Input: part model. Units: mm. Frame: model coordinates. A direction names the side the tool comes from. Coordinates: 2 decimals unless noted, no trailing zeros. Order: outer loops, then holes, each group sorted by start corner. A loop starts at its lowest first (then second) coordinate and runs counter-clockwise, first axis right, second up. Notation, with made-up numbers: (-19.5, -20) - (19.5, -20) arc R18 ccw to (19.5, 2) - close; hole circle Ø1 at (89, 45.25). An arc over 180 degrees is marked (long way). Use a Markdown table: item, result. Add a question column.
from build123d import *

# Parameters (mm, degrees)
SKETCH1_R           = 2.4892
BOSS_EXTRUDE1_DEPTH = 2.286
FILLET1_R           = 5.08


with BuildPart() as part:
    # Sketch1 → Boss-Extrude1 (new body)
    with BuildSketch(Plane.XY):
        with BuildLine():
            ThreePointArc((-10.16, 0), (-8.672102448, -3.592102448), (-5.08, -5.08))
            Line((-5.08, -5.08), (30.48, -5.08))
            ThreePointArc((30.48, -5.08), (34.072102448, -3.592102448), (35.56, 0))
            Line((35.56, 0), (35.56, 279.0825))
            ThreePointArc((35.56, 279.0825), (34.072102448, 282.674602448), (30.48, 284.1625))
            Line((30.48, 284.1625), (-5.08, 284.1625))
            ThreePointArc((-5.08, 284.1625), (-8.672102448, 282.674602448), (-10.16, 279.0825))
            Line((-10.16, 279.0825), (-10.16, 0))
        make_face()
        Circle(SKETCH1_R, mode=Mode.SUBTRACT)
        with BuildLine():
            Line((9.702242909, 36.253036461), (20.782825554, 11.949932204))
            ThreePointArc((20.782825554, 11.949932204), (20.433295811, 7.094715037), (16.160582646, 4.7625))
            Line((16.160582646, 4.7625), (5.08, 4.7625))
            ThreePointArc((5.08, 4.7625), (1.487897552, 6.250397552), (0, 9.8425))
            Line((0, 9.8425), (0, 34.145604258))
            ThreePointArc((0, 34.145604258), (4.001712927, 39.109846092), (9.702242909, 36.253036461))
        make_face(mode=Mode.SUBTRACT)
        with BuildLine():
            Line((0, 107.618145742), (0, 131.92125))
            ThreePointArc((0, 131.92125), (1.487897552, 135.513352448), (5.08, 137.00125))
            Line((5.08, 137.00125), (16.160582646, 137.00125))
            ThreePointArc((16.160582646, 137.00125), (20.433295811, 134.669034963), (20.782825554, 129.813817796))
            Line((20.782825554, 129.813817796), (9.702242909, 105.510713539))
            ThreePointArc((9.702242909, 105.510713539), (4.001712927, 102.653903908), (0, 107.618145742))
        make_face(mode=Mode.SUBTRACT)
        with Locations((25.4, 0)):
            Circle(SKETCH1_R, mode=Mode.SUBTRACT)
        with BuildLine():
            Line((15.697757091, 35.348465054), (0.457757091, 68.774442796))
            ThreePointArc((0.457757091, 68.774442796), (0, 70.881875), (0.457757091, 72.989307204))
            Line((0.457757091, 72.989307204), (15.697757091, 106.415284946))
            ThreePointArc((15.697757091, 106.415284946), (21.398287073, 109.272094577), (25.4, 104.307852743))
            Line((25.4, 104.307852743), (25.4, 37.455897257))
            ThreePointArc((25.4, 37.455897257), (21.398287073, 32.491655423), (15.697757091, 35.348465054))
        make_face(mode=Mode.SUBTRACT)
        with BuildLine():
            Line((0, 147.16125), (0, 171.464354258))
            ThreePointArc((0, 171.464354258), (4.001712927, 176.428596092), (9.702242909, 173.571786461))
            Line((9.702242909, 173.571786461), (20.782825554, 149.268682204))
            ThreePointArc((20.782825554, 149.268682204), (20.433295811, 144.413465037), (16.160582646, 142.08125))
            Line((16.160582646, 142.08125), (5.08, 142.08125))
            ThreePointArc((5.08, 142.08125), (1.487897552, 143.569147552), (0, 147.16125))
        make_face(mode=Mode.SUBTRACT)
        with BuildLine():
            ThreePointArc((0.457757091, 206.093192796), (0.115758165, 207.122337929), (0, 208.200625004))
            ThreePointArc((0, 208.200625004), (0.115758166, 209.278912075), (0.457757091, 210.308057204))
            Line((0.457757091, 210.308057204), (15.697757091, 243.734034946))
            ThreePointArc((15.697757091, 243.734034946), (21.398287073, 246.590844577), (25.4, 241.626602743))
            Line((25.4, 241.626602743), (25.4, 174.774647257))
            ThreePointArc((25.4, 174.774647257), (21.398287073, 169.810405423), (15.697757091, 172.667215054))
            Line((15.697757091, 172.667215054), (0.457757091, 206.093192796))
        make_face(mode=Mode.SUBTRACT)
        with Locations((0, 279.4)):
            Circle(SKETCH1_R, mode=Mode.SUBTRACT)
        with BuildLine():
            Line((5.08, 274.32), (16.160582646, 274.32))
            ThreePointArc((16.160582646, 274.32), (20.433295811, 271.987784963), (20.782825554, 267.132567796))
            Line((20.782825554, 267.132567796), (9.702242909, 242.829463539))
            ThreePointArc((9.702242909, 242.829463539), (4.001712927, 239.972653908), (0, 244.936895742))
            Line((0, 244.936895742), (0, 269.24))
            Line((0, 269.24), (0, 274.32))
            Line((0, 274.32), (5.08, 274.32))
        make_face(mode=Mode.SUBTRACT)
        with Locations((25.4, 279.4)):
            Circle(SKETCH1_R, mode=Mode.SUBTRACT)
    extrude(amount=BOSS_EXTRUDE1_DEPTH)

    # Fillet1
    fillet1_edges = [part.edges().sort_by_distance(p)[0] for p in [
        (0, 274.32, 1.143),
    ]]
    fillet(fillet1_edges, radius=FILLET1_R)


solid = part.part
1) Pull-direction query (Y, two-part tool) for faces 1 (the cylindrical face through (-8.711, -3.552, 1.127)), 2 (the cylindrical face through (4.096, 239.953, 1.127)), 3 (the cylindrical face through (-8.632, 282.714, 1.127)); classes: pulls with the +Y half, pulls with the -Y half, needs draft (parallel to the pull), parting line crosses it, or undercut.
2) Cut plane C-C (y = 194). Return the cut outline in (x, z).
3) Material intervals for L1, parallel to X at y = 279.4, z = 1.1; L2, parallel to Y at x = 24.5, z = 0.8; L3, parallel to Y at x = 27, z = 0.7, sorted ascending.
4) Contact query for flat-ended pins moving along their axis: P1, Ø3, axis at x = 25.4, y = 0, coming from the -Z side; P2, Ø2, axis at x = -3.5, y = 42.5, coming from the -Z side. Output: stop coordinate, or through.
5) Cut plane A-A (y = 16). Return the cut outline in (x, z).
6) Cut plane B-B (z = 1.15). State how many separate pieces and enclosed holes the cut face has, and give its area (3 significant figures).
7) Reachability of faces 4 (the cylindrical face through (34.032, -3.631, 1.127)), 5 (the cylindrical face through (1.53, 6.21, 1.13)) from +Z, -Z, +X, -X, +Y, -Y: full face, straight path, thin tool, end or side. Return the list, or none.
Computed:
| question | item | result |
|---|---|---|
| 1 | face 1 | pulls with the -Y half |
| 1 | face 2 | undercut |
| 1 | face 3 | pulls with the +Y half |
| 2 | outline | (-10.16, 0) - (5.97, 0) - (5.97, 2.29) - (-10.16, 2.29) - close; (25.4, 0) - (35.56, 0) - (35.56, 2.29) - (25.4, 2.29) - close |
| 3 | L1 | x = -10.15 to -2.49, 2.49 to 22.91, 27.89 to 35.55 |
| 3 | L2 | y = -5.08 to -2.32, 2.32 to 34.57, 107.19 to 171.89, 244.51 to 277.08, 281.72 to 284.16 |
| 3 | L3 | y = -5.08 to -1.91, 1.91 to 277.49, 281.31 to 284.16 |
| 4 | P1 | passes through |
| 4 | P2 | stops at z = 0 |
| 5 | outline | (-10.16, 0) - (0, 0) - (0, 2.29) - (-10.16, 2.29) - close; (18.94, 0) - (35.56, 0) - (35.56, 2.29) - (18.94, 2.29) - close |
| 6 | separate pieces | 1 |
| 6 | enclosed holes | 10 |
| 6 | area | 8,390 mm2 |
| 7 | face 4 | +Z, -Z, +X, -Y |
| 7 | face 5 | +Z, -Z |
